Input: part model. Units: mm. Frame: model coordinates. Coordinates: 2 decimals unless noted, no trailing zeros. Loops run counter-clockwise (first coordinate to the right, second up) from the corner with the lowest first, then second, coordinate; pieces in that order, holes last.
(1) Section A-A, the plane x = 0. Return loops of the section in (y, z), then the cut area to 3 significant figures.
(2) Line query: L1, parallel to X at y = -35.5, z = -2; L2, parallel to Y at x = -26.5, z = 0.4; L3, parallel to X at y = 10, z = 0.1. Output: solid intervals per line, ascending.
(3) Contact query for flat-ended pins moving along their axis: P1, Ø3, axis at x = -11.875, y = 22.875, coming from the +Z side; P2, Ø3, axis at y = -14, z = 1, coming from the -X side. Output: stop coordinate, or through.
(4) Section D-D, the plane y = 4. Return loops of the section in (x, z), then the cut area to 3 significant figures.
(5) Section C-C, the plane x = 12.5. Return loops of the section in (y, z).
(6) Section B-B, the plane y = 40. Return loops of the section in (x, z).
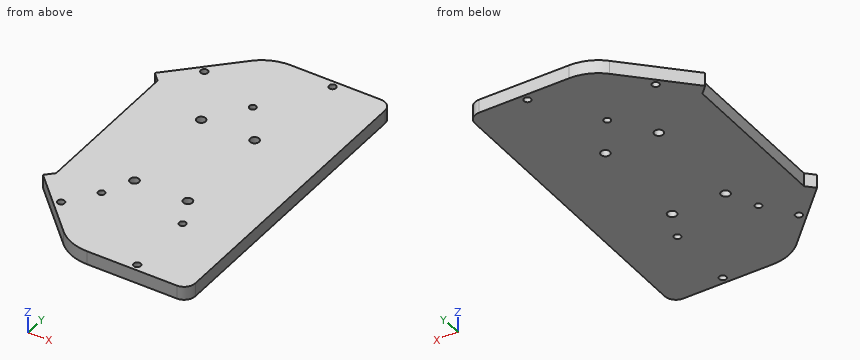
Solid Edge part; units mm, degrees
sketch "Sketch1" plane through (0, 0, 0) normal (0, 0, 1) x (1, 0, 0)
  line L0 (-2.5368, 70) -> (42.4632, 70)
  line L1 (42.4632, 70) -> (42.4632, -70)
  line L2 (-2.5368, -70) -> (42.4632, -70)
  arc A0 (-16.6789, -64.1421) -> (-2.5368, -70) centre (-2.5368, -50) ccw
  line L3 (-42.4632, -38.3579) -> (-16.6789, -64.1421)
  line L4 (-42.4632, -38.3579) -> (-38.9277, -34.8223)
  line L5 (-38.9277, 34.8223) -> (-38.9277, -34.8223)
  line L6 (-42.4632, 38.3579) -> (-38.9277, 34.8223)
  line L7 (-42.4632, 38.3579) -> (-16.6789, 64.1421)
  arc A1 (-16.6789, 64.1421) -> (-2.5368, 70) centre (-2.5368, 50) cw
  circle A2 centre (-27.4497, 49.1287) radius 1.5625
  circle A3 centre (17.9289, 67) radius 1.5625
  circle A4 centre (-27.4497, -49.1287) radius 1.5625
  circle A5 centre (17.9289, -67) radius 1.5625
extrude "Protrusion1" add sketch "Sketch1" along normal mid plane 6
fillet "Round_1" radius 5 2 edges at (42.4632, -70, 0) (42.4632, 70, 0)
sketch "Sketch2" plane through (0, 0, 3) normal (0, 0, 1) x (1, 0, 0)
  circle A0 centre (18, -36) radius 1.5
  circle A1 centre (-18, -36) radius 1.5
  circle A2 centre (0, 40) radius 1.5
  circle A3 centre (11.875, 22.875) radius 2
  circle A4 centre (11.875, -22.875) radius 2
  circle A5 centre (-11.875, -22.875) radius 2
  circle A6 centre (-11.875, 22.875) radius 2
extrude "ExtrudedCutout_1" cut sketch "Sketch2" against normal blind 7
Report:
1. outline: (-70, -3) - (38.5, -3) - (38.5, 3) - (-70, 3) - close; (41.5, -3) - (70, -3) - (70, 3) - (41.5, 3) - close
1. area: 822 mm2
2. L1: x = -39.61 to -19.41, -16.59 to 16.59, 19.41 to 42.46
2. L2: y = -54.32 to -50.37, -47.89 to 47.89, 50.37 to 54.32
2. L3: x = -38.93 to 42.46
3. P1: passes through
3. P2: stops at x = -38.93
4. outline: (-38.93, -3) - (42.46, -3) - (42.46, 3) - (-38.93, 3) - close
4. area: 488 mm2
5. outline: (-70, -3) - (-24.77, -3) - (-24.77, 3) - (-70, 3) - close; (-20.98, -3) - (20.98, -3) - (20.98, 3) - (-20.98, 3) - close; (24.77, -3) - (70, -3) - (70, 3) - (24.77, 3) - close
6. outline: (-40.82, -3) - (-1.5, -3) - (-1.5, 3) - (-40.82, 3) - close; (1.5, -3) - (42.46, -3) - (42.46, 3) - (1.5, 3) - close
